Model file for the job. Use its own axes, mm. Face numbers are marked on the shaded views. A direction names the side the tool comes from. Give positions to 0.01 mm unless a question says otherwise; leave off trailing zeros. Order: outer loops, then holes, each group sorted by start corner. A loop starts at its lowest first (then second) coordinate and runs counter-clockwise, first axis right, second up. Notation, with made-up numbers: M 46,41 L 78,41 A26 cw 78,73 Z; hole C 79.5,34.25 d6. An arc over 180 degrees is marked long. Return JSON: item names as keys, results as strings. Group by question number.
1. Pin check, flat tips, straight feed: pin 1 (3 mm diameter, centred on x = -16.2, z = -18.2, fed in from +Y); pin 2 (1.2 mm diameter, centred on x = 9, z = -22.5, fed in from +Y). Stop position of each tip, or through.
2. Slice it at A-A on x = 6. List the corners of the cut face in (y, z), then the cut area to 3 significant figures.
3. 3-axis set-ups, long thin cutter, end or side, ignore diameter. For the marked faces 1 and 2: which of +Z, -Z, +X, -X, +Y, -Y reach the whole face in a straight line?
4. Slice it at C-C on y = -10.5. List the corners of the cut face in (x, z), then the cut area to 3 significant figures.
5. Wall check: probe 1 along Z at (x, y) = (-16.2, -13.25); probe 2 along Y at (x, z) = (-16.2, -22.25); probe 3 along Z at (x, y) = (11.5, -13). Give the ranges that are in metal, low to high. Write a range as [from, to].
6. Slice it at B-B on z = -11. List the corners of the cut face in (x, y), then the cut area to 3 significant figures.
7. Slice it at D-D on z = -3.8. List the corners of the cut face in (x, y), then the cut area to 3 significant figures.
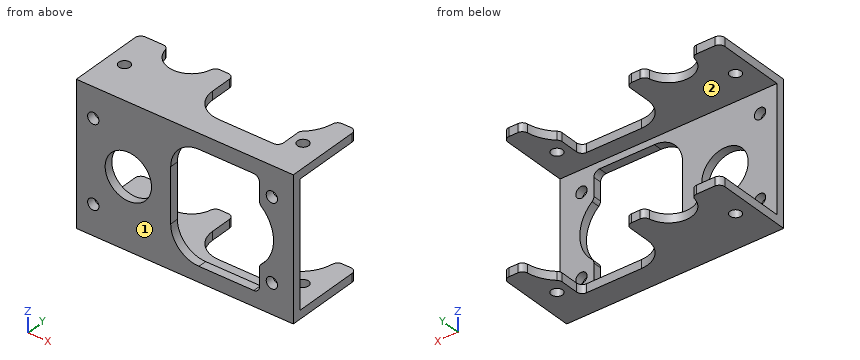
from build123d import *

# Parameters (mm, degrees)
F0_W     = 38.4
F0_H     = 28.4
F0_R     = 1
F0_R_2   = 4.1
F1_DEPTH = 1.5
F2_W     = 38.4
F2_H     = 1.5
F3_DEPTH = 22
F6_W     = 38.4
F6_H     = 14.2
F7_DEPTH = 25.001
F8_R     = 4.1
F8_R_2   = 1
F9_DEPTH = 1.5
F10_R    = 1


with BuildPart() as f1:
    # F0 (on Top) → F1 (new body)
    with BuildSketch(Plane.XY):
        Rectangle(F0_W, F0_H)
        with Locations((-16.2, -7.2)):
            Circle(F0_R, mode=Mode.SUBTRACT)
        with Locations((15.4, -7.2)):
            Circle(F0_R, mode=Mode.SUBTRACT)
        with Locations((-10, 0)):
            Circle(F0_R_2, mode=Mode.SUBTRACT)
        with Locations((-16.2, 7.2)):
            Circle(F0_R, mode=Mode.SUBTRACT)
        with BuildLine():
            ThreePointArc((-2.5, 4.8), (-1.0355339059, 8.3355339059), (2.5, 9.8))
            Line((2.5, 9.8), (12.2, 9.8))
            ThreePointArc((12.2, 9.8), (12.9071067812, 9.5071067812), (13.2, 8.8))
            Line((13.2, 8.8), (13.2, 5.5901699437))
            ThreePointArc((13.2, 5.5901699437), (13.2871290708, 5.1819216533), (13.5333333333, 4.8448139512))
            ThreePointArc((13.5333333333, 4.8448139512), (15.7, 0), (13.5333333333, -4.8448139512))
            ThreePointArc((13.5333333333, -4.8448139512), (13.2871290708, -5.1819216533), (13.2, -5.5901699437))
            Line((13.2, -5.5901699437), (13.2, -8.8))
            ThreePointArc((13.2, -8.8), (12.9071067812, -9.5071067812), (12.2, -9.8))
            Line((12.2, -9.8), (2.5, -9.8))
            ThreePointArc((2.5, -9.8), (-1.0355339059, -8.3355339059), (-2.5, -4.8))
            Line((-2.5, -4.8), (-2.5, 4.8))
        make_face(mode=Mode.SUBTRACT)
        with Locations((15.4, 7.2)):
            Circle(F0_R, mode=Mode.SUBTRACT)
    extrude(amount=F1_DEPTH)

    # F2 (on face) → F3 (join)
    with BuildSketch(Plane(origin=(0, 0, 0), x_dir=(1, 0, 0), z_dir=(0, 0, -1))):
        with Locations((0, 13.45)):
            Rectangle(F2_W, F2_H)
    extrude(amount=F3_DEPTH)

    # F5: F1 across plane


with BuildPart() as f1_1:
    add(f1.part)
    add(f1.part.mirror(Plane.XY.offset(-11)))

    # F6 (on face) → F7 (cut, through all)
    with BuildSketch(Plane(origin=(0, 0, -23.5), x_dir=(1, 0, 0), z_dir=(0, 0, -1))):
        with Locations((0, -7.1)):
            Rectangle(F6_W, F6_H)
    extrude(amount=-F7_DEPTH, mode=Mode.SUBTRACT)

    # F8 (on face) → F9 (cut, through all)
    with BuildSketch(Plane.XZ.offset(14.2)):
        with Locations((-10, -11)):
            Circle(F8_R)
        with Locations((-16.2, -3.8)):
            Circle(F8_R_2)
        with Locations((15.4, -3.8)):
            Circle(F8_R_2)
        with BuildLine():
            Line((12.2, -1.2), (2.5, -1.2))
            ThreePointArc((2.5, -1.2), (-1.0355339059, -2.6644660941), (-2.5, -6.2))
            Line((-2.5, -6.2), (-2.5, -15.8))
            ThreePointArc((-2.5, -15.8), (-1.0355339059, -19.3355339059), (2.5, -20.8))
            Line((2.5, -20.8), (12.2, -20.8))
            ThreePointArc((12.2, -20.8), (12.9071067812, -20.5071067812), (13.2, -19.8))
            Line((13.2, -19.8), (13.2, -16.5901699437))
            ThreePointArc((13.2, -16.5901699437), (13.2871290708, -16.1819216533), (13.5333333333, -15.8448139512))
            ThreePointArc((13.5333333333, -15.8448139512), (15.7, -11), (13.5333333333, -6.1551860488))
            ThreePointArc((13.5333333333, -6.1551860488), (13.2871290708, -5.8180783467), (13.2, -5.4098300563))
            Line((13.2, -5.4098300563), (13.2, -2.2))
            ThreePointArc((13.2, -2.2), (12.9071067812, -1.4928932188), (12.2, -1.2))
        make_face()
        with Locations((-16.2, -18.2)):
            Circle(F8_R_2)
        with Locations((15.4, -18.2)):
            Circle(F8_R_2)
    extrude(amount=-F9_DEPTH, mode=Mode.SUBTRACT)

    # F10
    f10_edges = [f1_1.edges().sort_by_distance(p)[0] for p in [
        (-19.2, 0, -22.75),
        (-19.2, 0, 0.75),
        (-5.9, 0, 0.75),
        (-14.1, 0, 0.75),
        (-5.9, 0, -22.75),
        (-14.1, 0, -22.75),
        (-2.5, 0, -22.75),
        (15.7, 0, -22.75),
        (15.7, 0, 0.75),
        (19.2, 0, -22.75),
        (19.2, 0, 0.75),
        (-2.5, 0, 0.75),
    ]]
    fillet(f10_edges, radius=F10_R)


solid = f1_1.part
Result:
{
 "1": {"pin 1": "stops at y = -12.7", "pin 2": "stops at y = -9.8"},
 "2": {"outline": "M -14.2,-23.5 L -9.8,-23.5 L -9.8,-22 L -12.7,-22 L -12.7,-20.8 L -14.2,-20.8 Z; M -14.2,-1.2 L -12.7,-1.2 L -12.7,0 L -9.8,0 L -9.8,1.5 L -14.2,1.5 Z", "area": "16.8 mm2"},
 "3": {"face 1": "+Z, -Z, +X, -X, -Y", "face 2": "+X, -X, +Y"},
 "4": {"outline": "M -19.2,-23.5 L 19.2,-23.5 L 19.2,-22 L -19.2,-22 Z; M -19.2,0 L 19.2,0 L 19.2,1.5 L -19.2,1.5 Z", "area": "115 mm2"},
 "5": {"probe 1": "z = [-23.5, -19.2], [-17.2, -4.8], [-2.8, 1.5]", "probe 2": "y = [-14.2, -8.2], [-6.2, 0]", "probe 3": "z = [-23.5, -20.8], [-1.2, 1.5]"},
 "6": {"outline": "M -19.2,-14.2 L -14.1,-14.2 L -14.1,-12.7 L -19.2,-12.7 Z; M -5.9,-14.2 L -2.5,-14.2 L -2.5,-12.7 L -5.9,-12.7 Z; M 15.7,-14.2 L 19.2,-14.2 L 19.2,-12.7 L 15.7,-12.7 Z", "area": "18.0 mm2"},
 "7": {"outline": "M -19.2,-14.2 L -17.2,-14.2 L -17.2,-12.7 L -19.2,-12.7 Z; M -15.2,-14.2 L -1.89,-14.2 L -1.89,-12.7 L -15.2,-12.7 Z; M 13.2,-14.2 L 14.4,-14.2 L 14.4,-12.7 L 13.2,-12.7 Z; M 16.4,-14.2 L 19.2,-14.2 L 19.2,-12.7 L 16.4,-12.7 Z", "area": "29.0 mm2"}
}
